Here's how the part is built. I have some questions about the finished solid (model axes, mm). A direction names the side the tool comes from. Coordinates: 2 decimals unless noted, no trailing zeros. Order: outer loops, then holes, each group sorted by start corner. A loop starts at its lowest first (then second) coordinate and runs counter-clockwise, first axis right, second up. Notation, with made-up numbers: (-16.75, -23.75) -> (-7.75, -23.75) arc R17 cw to (-7.75, -9.75) -> close; hole circle Ø3 at (61, 7.25). An arc over 180 degrees is marked (long way). One line per item, written item: value. Start each with the question number.
```python
from build123d import *

# Parameters (mm, degrees)
BOSS_EXTRU_1_DEPTH      = 5
BOSS_EXTRU_2_DEPTH      = 2
ESQUISSE4_R             = 1.9
ENL_V_MAT_EXTRU_1_DEPTH = 5


with BuildPart() as part:
    # Esquisse2 → Boss.-Extru.1 (new body)
    with BuildSketch(Plane.XY):
        with BuildLine():
            Line((-5.621162791, 2.893255814), (-4.121162791, 2.893255814))
            Line((-4.121162791, 2.893255814), (-4.121162791, 0.093255814))
            ThreePointArc((-4.121162791, 0.093255814), (-3.974716181, -0.260297577), (-3.621162791, -0.406744186))
            Line((-3.621162791, -0.406744186), (20.378837209, -0.406744186))
            ThreePointArc((20.378837209, -0.406744186), (20.7323906, -0.260297577), (20.878837209, 0.093255814))
            Line((20.878837209, 0.093255814), (20.878837209, 2.893255814))
            Line((20.878837209, 2.893255814), (22.378837209, 2.893255814))
            Line((22.378837209, 2.893255814), (22.378837209, -0.965813953))
            ThreePointArc((22.378837209, -0.965813953), (22.2323906, -1.319367344), (21.878837209, -1.465813953))
            Line((21.878837209, -1.465813953), (-5.121162791, -1.465813953))
            ThreePointArc((-5.121162791, -1.465813953), (-5.474716181, -1.319367344), (-5.621162791, -0.965813953))
            Line((-5.621162791, -0.965813953), (-5.621162791, 2.893255814))
        make_face()
    extrude(amount=BOSS_EXTRU_1_DEPTH)

    # Esquisse3 → Boss.-Extru.2 (add)
    with BuildSketch(Plane(origin=(0, 2.893255814, 0), x_dir=(1, 0, 0), z_dir=(0, 1, 0))):
        with BuildLine():
            Line((-5.621162791, 0), (-10.121162791, 0))
            ThreePointArc((-10.121162791, 0), (-10.474716181, -0.146446609), (-10.621162791, -0.5))
            Line((-10.621162791, -0.5), (-10.621162791, -4.5))
            ThreePointArc((-10.621162791, -4.5), (-10.474716181, -4.853553391), (-10.121162791, -5))
            Line((-10.121162791, -5), (-5.621162791, -5))
            Line((-5.621162791, -5), (-5.621162791, 0))
        make_face()
        with BuildLine():
            Line((22.378837209, -5), (26.878837209, -5))
            ThreePointArc((26.878837209, -5), (27.2323906, -4.853553391), (27.378837209, -4.5))
            Line((27.378837209, -4.5), (27.378837209, -0.5))
            ThreePointArc((27.378837209, -0.5), (27.2323906, -0.146446609), (26.878837209, 0))
            Line((26.878837209, 0), (22.378837209, 0))
            Line((22.378837209, 0), (22.378837209, -5))
        make_face()
    extrude(amount=-BOSS_EXTRU_2_DEPTH)

    # Esquisse4 → Enlèv. mat.-Extru.1 (cut)
    with BuildSketch(Plane(origin=(0, 2.893255814, 0), x_dir=(1, 0, 0), z_dir=(0, 1, 0))):
        with Locations(Location((-8.153362247, -2.5, 0), (0, 0, 270))):
            Circle(ESQUISSE4_R)
        with Locations(Location((24.911036665, -2.5, 0), (0, 0, 270))):
            Circle(ESQUISSE4_R)
    extrude(amount=-ENL_V_MAT_EXTRU_1_DEPTH, mode=Mode.SUBTRACT)


solid = part.part
```
Q1. Imagine slicing it at C-C (x = -7.5). Write out the boundary of the cut face in (y, z).
Q2. I need wall thicknesses on line 1 (X direction, y = 1.5, z = 2.5); line 2 (X direction, y = 2.6, z = 0.9); line 3 (X direction, y = 0.3, z = 0.45). Which ranges of each line are inside material? Lowest first, please.
Q3. Imagine slicing it at A-A (z = 2.5). Write out the boundary of the cut face in (x, y).
Q4. If we mould it in two halves opening along X, with no side actions, what happens to faces 1 (the face through (-10.621, 2, 2)), 2 (the face through (20.879, 1, 2)), 3 (the face through (27.379, 2, 3)), 4 (the face through (-7, 0.893, 0.8))? For each: +X half, -X half, draft (parallel to the pull), parting line (faces both ways), or undercut.
Q5. Imagine slicing it at B-B (y = 2.4). Write out the boundary of the cut face in (x, z), plus the area to 3 significant figures.
Q6. For faces 5 (the face through (-5.621, 0, 2)), 6 (the face through (-4.121, 2, 2)), 7 (the face through (8, -1, 5)), 8 (the face through (27, 0.893, 1)), 9 (the face through (-9.839, 1.907, 3.377)), which set-ups out of +Z, -Z, +X, -X, +Y, -Y let a thin tool reach every point of the face, with its end or its side?
Q7. For P1, Ø0.9, axis at y = -0.5, z = 2.5, coming from the -X side; P2, Ø1.5, axis at x = 8, z = 2.5, coming from the +Y side; P3, Ø0.6, axis at y = 0, z = 3.5, coming from the +X side, each with a flat end and sliding along its axis, tell me the tip position at first contact or that it passes through.
Q8. Imagine slicing it at D-D (x = 19.5). Write out the boundary of the cut face in (y, z), plus the area to 3 significant figures.
Completed:
1. outline: (0.89, 0) -> (2.89, 0) -> (2.89, 0.72) -> (0.89, 0.72) -> close; (0.89, 4.28) -> (2.89, 4.28) -> (2.89, 5) -> (0.89, 5) -> close
2. line 1: x = -10.62 to -10.05, -6.25 to -4.12, 20.88 to 23.01, 26.81 to 27.38
2. line 2: x = -10.62 to -9.18, -7.13 to -4.12, 20.88 to 23.89, 25.94 to 27.38
2. line 3: x = -5.62 to -4.12, 20.88 to 22.38
3. outline: (-10.62, 0.89) -> (-10.05, 0.89) -> (-10.05, 2.89) -> (-10.62, 2.89) -> close; (-6.25, 0.89) -> (-5.62, 0.89) -> (-5.62, -0.97) arc R0.5 ccw to (-5.12, -1.47) -> (21.88, -1.47) arc R0.5 ccw to (22.38, -0.97) -> (22.38, 0.89) -> (23.01, 0.89) -> (23.01, 2.89) -> (20.88, 2.89) -> (20.88, 0.09) arc R0.5 cw to (20.38, -0.41) -> (-3.62, -0.41) arc R0.5 cw to (-4.12, 0.09) -> (-4.12, 2.89) -> (-6.25, 2.89) -> close; (26.81, 0.89) -> (27.38, 0.89) -> (27.38, 2.89) -> (26.81, 2.89) -> close
4. face 1: -X half
4. face 2: undercut
4. face 3: +X half
4. face 4: draft
5. outline: (-10.62, 0.5) arc R0.5 ccw to (-10.12, 0) -> (-4.12, 0) -> (-4.12, 5) -> (-10.12, 5) arc R0.5 ccw to (-10.62, 4.5) -> close; (20.88, 0) -> (26.88, 0) arc R0.5 ccw to (27.38, 0.5) -> (27.38, 4.5) arc R0.5 ccw to (26.88, 5) -> (20.88, 5) -> close; hole circle Ø3.8 at (-8.15, 2.5); hole circle Ø3.8 at (24.91, 2.5)
5. area: 42.1 mm2
6. face 5: +Z, -Z, -X, -Y
6. face 6: +Z, -Z, +Y
6. face 7: +Z, +X, -X, +Y, -Y
6. face 8: +Z, -Z, +X, -Y
6. face 9: +Y, -Y
7. P1: stops at x = -5.62
7. P2: stops at y = -0.41
7. P3: stops at x = 22.38
8. outline: (-1.47, 0) -> (-0.41, 0) -> (-0.41, 5) -> (-1.47, 5) -> close
8. area: 5.30 mm2
